The listing builds one solid part. Answer for the finished solid, in the listing's coordinates (mm). A direction names the side the tool comes from. Give positions to 0.01 mm unless a question says otherwise; leave off trailing zeros. Write each loop counter-clockwise with the first axis right and the second up, starting at its lowest first coordinate (ties: lowest second). Pieces come first, ordered by that corner, then holes. Notation, with made-up numbers: (77.5, 76.5) - (89.5, 76.5) arc R29 cw to (89.5, 108.5) - close; hole circle Ø5 at (16, -2). An arc over 180 degrees is marked (long way). Use a Markdown table: item, result. Add a question column.
from build123d import *

# Parameters (mm, degrees)
SKETCH_1_W          = 241
SKETCH_1_H          = 92
EXTRUDE_1_DEPTH     = 2
FILLET_1_R          = 5
FILLET_2_R          = 11
CUT_EXTRUDE_1_REACH = 130.997
SKETCH_3_R          = 1
SKETCH_4_R          = 2
CUT_EXTRUDE_2_DEPTH = 1.3
EXTRUDE_START       = 2
EXTRUDE_2_DEPTH     = 2
CHAMFER_1_SIZE      = 0.174977327
CHAMFER_1_SIZE_2    = 2
SKETCH_6_W          = 5
SKETCH_6_H          = 85
EXTRUDE_3_DEPTH     = 6.3
CUT_EXTRUDE_3_REACH = 131.135
SKETCH_7_W          = 21
SKETCH_7_H          = 60
EXTRUDE_START_2     = -28.5
EXTRUDE_4_DEPTH     = 2
CHAMFER_2_SIZE      = 3
CHAMFER_2_SIZE2     = 1.732050808


with BuildPart() as part:
    # 草图1 → 凸台-拉伸1 (new body)
    with BuildSketch(Plane.XY):
        Rectangle(SKETCH_1_W, SKETCH_1_H)
    extrude(amount=EXTRUDE_1_DEPTH)

    # 圆角1
    fillet_1_edges = [part.edges().sort_by_distance(p)[0] for p in [
        (-120.5, -46, 1),
    ]]
    fillet(fillet_1_edges, radius=FILLET_1_R)

    # 圆角2
    fillet_2_edges = [part.edges().sort_by_distance(p)[0] for p in [
        (120.5, -46, 1),
        (-120.5, 46, 1),
        (120.5, 46, 1),
    ]]
    fillet(fillet_2_edges, radius=FILLET_2_R)

    # 草图3 → 切除-拉伸1 (cut, up to next)
    with BuildSketch(Plane.XY.offset(2), mode=Mode.PRIVATE) as cut_extrude_1_sk1:
        with Locations((-19.5, -41)):
            Circle(SKETCH_3_R)
    cut_extrude_1_tool1 = extrude(cut_extrude_1_sk1.sketch, amount=-CUT_EXTRUDE_1_REACH, mode=Mode.PRIVATE) & part.part
    # 草图3 → 切除-拉伸1 (cut, up to next)
    with BuildSketch(Plane.XY.offset(2), mode=Mode.PRIVATE) as cut_extrude_1_sk2:
        with Locations((-74.5, -40)):
            Circle(SKETCH_3_R)
    cut_extrude_1_tool2 = extrude(cut_extrude_1_sk2.sketch, amount=-CUT_EXTRUDE_1_REACH, mode=Mode.PRIVATE) & part.part
    # 草图3 → 切除-拉伸1 (cut, up to next)
    with BuildSketch(Plane.XY.offset(2), mode=Mode.PRIVATE) as cut_extrude_1_sk3:
        with Locations((-113.5, 39)):
            Circle(SKETCH_3_R)
    cut_extrude_1_tool3 = extrude(cut_extrude_1_sk3.sketch, amount=-CUT_EXTRUDE_1_REACH, mode=Mode.PRIVATE) & part.part
    # 草图3 → 切除-拉伸1 (cut, up to next)
    with BuildSketch(Plane.XY.offset(2), mode=Mode.PRIVATE) as cut_extrude_1_sk4:
        with Locations((0, 39)):
            Circle(SKETCH_3_R)
    cut_extrude_1_tool4 = extrude(cut_extrude_1_sk4.sketch, amount=-CUT_EXTRUDE_1_REACH, mode=Mode.PRIVATE) & part.part
    # 草图3 → 切除-拉伸1 (cut, up to next)
    with BuildSketch(Plane.XY.offset(2), mode=Mode.PRIVATE) as cut_extrude_1_sk5:
        with Locations((113.5, -39)):
            Circle(SKETCH_3_R)
    cut_extrude_1_tool5 = extrude(cut_extrude_1_sk5.sketch, amount=-CUT_EXTRUDE_1_REACH, mode=Mode.PRIVATE) & part.part
    # 草图3 → 切除-拉伸1 (cut, up to next)
    with BuildSketch(Plane.XY.offset(2), mode=Mode.PRIVATE) as cut_extrude_1_sk6:
        with Locations((113.5, 39)):
            Circle(SKETCH_3_R)
    cut_extrude_1_tool6 = extrude(cut_extrude_1_sk6.sketch, amount=-CUT_EXTRUDE_1_REACH, mode=Mode.PRIVATE) & part.part
    add(cut_extrude_1_tool1.solids().sort_by_distance((-19.5, -41, 2))[0], mode=Mode.SUBTRACT)
    add(cut_extrude_1_tool2.solids().sort_by_distance((-74.5, -40, 2))[0], mode=Mode.SUBTRACT)
    add(cut_extrude_1_tool3.solids().sort_by_distance((-113.5, 39, 2))[0], mode=Mode.SUBTRACT)
    add(cut_extrude_1_tool4.solids().sort_by_distance((0, 39, 2))[0], mode=Mode.SUBTRACT)
    add(cut_extrude_1_tool5.solids().sort_by_distance((113.5, -39, 2))[0], mode=Mode.SUBTRACT)
    add(cut_extrude_1_tool6.solids().sort_by_distance((113.5, 39, 2))[0], mode=Mode.SUBTRACT)

    # 草图4 → 切除-拉伸2 (cut)
    with BuildSketch(Plane(origin=(0, 0, 0), x_dir=(-1, 0, 0), z_dir=(0, 0, -1))):
        with Locations((74.5, -40)):
            Circle(SKETCH_4_R)
        with Locations((19.5, -41)):
            Circle(SKETCH_4_R)
        with Locations((-113.5, -39)):
            Circle(SKETCH_4_R)
        with Locations((-113.5, 39)):
            Circle(SKETCH_4_R)
        with Locations((0, 39)):
            Circle(SKETCH_4_R)
        with Locations((113.5, 39)):
            Circle(SKETCH_4_R)
    extrude(amount=-CUT_EXTRUDE_2_DEPTH, mode=Mode.SUBTRACT)

    # 草图5 → 凸台-拉伸2 (add)
    with BuildSketch(Plane.XY.offset(2).offset(EXTRUDE_START)):
        with BuildLine():
            ThreePointArc((-120.5, -41), (-119.035533906, -44.535533906), (-115.5, -46))
            Line((-115.5, -46), (109.5, -46))
            ThreePointArc((109.5, -46), (117.278174593, -42.778174593), (120.5, -35))
            Line((120.5, -35), (120.5, 35))
            ThreePointArc((120.5, 35), (117.278174593, 42.778174593), (109.5, 46))
            Line((109.5, 46), (-109.5, 46))
            ThreePointArc((-109.5, 46), (-117.278174593, 42.778174593), (-120.5, 35))
            Line((-120.5, 35), (-120.5, -41))
        make_face()
        with BuildLine():
            Line((109.5, -44.7), (-115.5, -44.7))
            ThreePointArc((-115.5, -44.7), (-118.11629509, -43.61629509), (-119.2, -41))
            Line((-119.2, -41), (-119.2, 35))
            ThreePointArc((-119.2, 35), (-116.358935778, 41.858935778), (-109.5, 44.7))
            Line((-109.5, 44.7), (109.5, 44.7))
            ThreePointArc((109.5, 44.7), (116.358935778, 41.858935778), (119.2, 35))
            Line((119.2, 35), (119.2, -35))
            ThreePointArc((119.2, -35), (116.358935778, -41.858935778), (109.5, -44.7))
        make_face(mode=Mode.SUBTRACT)
    extrude(amount=-EXTRUDE_2_DEPTH)

    # 倒角1
    # the kernel refuses this chamfer: 2, 0.174977327 mm, written as the material it takes off along each edge
    with BuildSketch(Plane(origin=(-109.5, 44.7, 4), x_dir=(0, 0.9159861691531133, 0.40120984275090293), z_dir=(1, 0, 0))) as chamfer_1_piece_1_section:
        Polygon((CHAMFER_1_SIZE * 0.915986169425, -CHAMFER_1_SIZE * 0.40120984287), (-CHAMFER_1_SIZE_2 * 0.401209842751, -CHAMFER_1_SIZE_2 * 0.915986169153), (0, 0), align=None)
    chamfer_1_piece_1 = extrude(amount=219, mode=Mode.PRIVATE)
    chamfer_1_piece_1 = split(chamfer_1_piece_1, bisect_by=Plane(origin=(0, 44.735649873, 2), z_dir=(0, 0, 1)), keep=Keep.TOP, mode=Mode.PRIVATE)
    add(chamfer_1_piece_1, mode=Mode.SUBTRACT)
    with BuildSketch(Plane(origin=(109.5, 35, 4), x_dir=(0, 1, 0), z_dir=(-1, 0, 0))) as chamfer_1_piece_2_section:
        Polygon((9.7 + CHAMFER_1_SIZE, 0), (9.7, CHAMFER_1_SIZE_2), (9.7, 0), align=None)
    chamfer_1_piece_2 = revolve(axis=Axis((109.5, 35, 4), (0, 0, -1)), revolution_arc=90, mode=Mode.PRIVATE)
    chamfer_1_piece_2 = split(chamfer_1_piece_2, bisect_by=Plane(origin=(116.41200817, 41.91200817, 2), z_dir=(0, 0, 1)), keep=Keep.TOP, mode=Mode.PRIVATE)
    add(chamfer_1_piece_2, mode=Mode.SUBTRACT)
    with BuildSketch(Plane(origin=(-109.5, 35, 4), x_dir=(-1, 0, 0), z_dir=(0, -1, 0))) as chamfer_1_piece_3_section:
        Polygon((9.7 + CHAMFER_1_SIZE, 0), (9.7, CHAMFER_1_SIZE_2), (9.7, 0), align=None)
    chamfer_1_piece_3 = revolve(axis=Axis((-109.5, 35, 4), (0, 0, -1)), revolution_arc=90, mode=Mode.PRIVATE)
    chamfer_1_piece_3 = split(chamfer_1_piece_3, bisect_by=Plane(origin=(-116.412008168, 41.912008168, 2), z_dir=(0, 0, 1)), keep=Keep.TOP, mode=Mode.PRIVATE)
    add(chamfer_1_piece_3, mode=Mode.SUBTRACT)
    with BuildSketch(Plane(origin=(119.2, 35, 4), x_dir=(0.9159861691531133, 0, 0.40120984275090293), z_dir=(0, -1, 0))) as chamfer_1_piece_4_section:
        Polygon((CHAMFER_1_SIZE * 0.915986169425, -CHAMFER_1_SIZE * 0.40120984287), (-CHAMFER_1_SIZE_2 * 0.401209842751, -CHAMFER_1_SIZE_2 * 0.915986169153), (0, 0), align=None)
    chamfer_1_piece_4 = extrude(amount=70, mode=Mode.PRIVATE)
    chamfer_1_piece_4 = split(chamfer_1_piece_4, bisect_by=Plane(origin=(119.235649873, 0, 2), z_dir=(0, 0, 1)), keep=Keep.TOP, mode=Mode.PRIVATE)
    add(chamfer_1_piece_4, mode=Mode.SUBTRACT)
    with BuildSketch(Plane(origin=(-119.2, -41, 4), x_dir=(-0.9159861691531133, 0, 0.40120984275090293), z_dir=(0, 1, 0))) as chamfer_1_piece_5_section:
        Polygon((CHAMFER_1_SIZE * 0.915986169425, -CHAMFER_1_SIZE * 0.40120984287), (-CHAMFER_1_SIZE_2 * 0.401209842751, -CHAMFER_1_SIZE_2 * 0.915986169153), (0, 0), align=None)
    chamfer_1_piece_5 = extrude(amount=76, mode=Mode.PRIVATE)
    chamfer_1_piece_5 = split(chamfer_1_piece_5, bisect_by=Plane(origin=(-119.235649873, -3, 2), z_dir=(0, 0, 1)), keep=Keep.TOP, mode=Mode.PRIVATE)
    add(chamfer_1_piece_5, mode=Mode.SUBTRACT)
    with BuildSketch(Plane(origin=(109.5, -35, 4), x_dir=(1, 0, 0), z_dir=(0, 1, 0))) as chamfer_1_piece_6_section:
        Polygon((9.7 + CHAMFER_1_SIZE, 0), (9.7, CHAMFER_1_SIZE_2), (9.7, 0), align=None)
    chamfer_1_piece_6 = revolve(axis=Axis((109.5, -35, 4), (0, 0, -1)), revolution_arc=90, mode=Mode.PRIVATE)
    chamfer_1_piece_6 = split(chamfer_1_piece_6, bisect_by=Plane(origin=(116.41200817, -41.91200817, 2), z_dir=(0, 0, 1)), keep=Keep.TOP, mode=Mode.PRIVATE)
    add(chamfer_1_piece_6, mode=Mode.SUBTRACT)
    with BuildSketch(Plane(origin=(-115.5, -41, 4), x_dir=(0, -1, 0), z_dir=(1, 0, 0))) as chamfer_1_piece_7_section:
        Polygon((3.7 + CHAMFER_1_SIZE, 0), (3.7, CHAMFER_1_SIZE_2), (3.7, 0), align=None)
    chamfer_1_piece_7 = revolve(axis=Axis((-115.5, -41, 4), (0, 0, -1)), revolution_arc=90, mode=Mode.PRIVATE)
    chamfer_1_piece_7 = split(chamfer_1_piece_7, bisect_by=Plane(origin=(-118.172444307, -43.672444307, 2), z_dir=(0, 0, 1)), keep=Keep.TOP, mode=Mode.PRIVATE)
    add(chamfer_1_piece_7, mode=Mode.SUBTRACT)
    with BuildSketch(Plane(origin=(109.5, -44.7, 4), x_dir=(0, -0.9159861691531133, 0.40120984275090293), z_dir=(-1, 0, 0))) as chamfer_1_piece_8_section:
        Polygon((CHAMFER_1_SIZE * 0.915986169425, -CHAMFER_1_SIZE * 0.40120984287), (-CHAMFER_1_SIZE_2 * 0.401209842751, -CHAMFER_1_SIZE_2 * 0.915986169153), (0, 0), align=None)
    chamfer_1_piece_8 = extrude(amount=225, mode=Mode.PRIVATE)
    chamfer_1_piece_8 = split(chamfer_1_piece_8, bisect_by=Plane(origin=(-3, -44.735649873, 2), z_dir=(0, 0, 1)), keep=Keep.TOP, mode=Mode.PRIVATE)
    add(chamfer_1_piece_8, mode=Mode.SUBTRACT)

    # 草图6 → 凸台-拉伸3 (add)
    with BuildSketch(Plane.XY.offset(2)):
        with Locations((26.5, 0)):
            Rectangle(SKETCH_6_W, SKETCH_6_H)
    extrude(amount=EXTRUDE_3_DEPTH)

    # 草图7 → 切除-拉伸3 (cut, up to next)
    with BuildSketch(Plane.XY.offset(2), mode=Mode.PRIVATE) as cut_extrude_3_sk1:
        with Locations((-104.5, -9)):
            Rectangle(SKETCH_7_W, SKETCH_7_H)
    cut_extrude_3_tool1 = extrude(cut_extrude_3_sk1.sketch, amount=-CUT_EXTRUDE_3_REACH, mode=Mode.PRIVATE) & part.part
    add(cut_extrude_3_tool1.solids().sort_by_distance((-104.5, -9, 2))[0], mode=Mode.SUBTRACT)

    # 草图8 → 凸台-拉伸4 (add)
    with BuildSketch(Plane.ZY.offset(120.5).offset(EXTRUDE_START_2)):
        with BuildLine():
            Line((2, -21), (2, -42.5))
            Line((2, -42.5), (39.5, -42.5))
            Line((39.5, -42.5), (39.5, -40.556496954))
            ThreePointArc((39.5, -40.556496954), (19.774984647, -36.291232599), (6.605059959, -21))
            Line((6.605059959, -21), (2, -21))
        make_face()
        with BuildLine():
            Line((2, -14), (4.646172482, -14))
            ThreePointArc((4.646172482, -14), (5.952882138, 1.25832385), (14.25, 14.130067012))
            Line((14.25, 14.130067012), (14.25, 27))
            Line((14.25, 27), (12.5, 27))
            Line((12.5, 27), (12.5, 42.479565739))
            Line((12.5, 42.479565739), (2, 42.479565739))
            Line((2, 42.479565739), (2, -14))
        make_face()
    extrude(amount=EXTRUDE_4_DEPTH)

    # 倒角2
    chamfer_2_edges = [part.edges().sort_by_distance(p)[0] for p in [
        (-104.5, -39, 0),
        (-115, -9, 0),
        (-104.5, 21, 0),
        (-94, -9, 0),
    ]]
    chamfer_2_side = [part.faces().sort_by_distance(p)[0] for p in [
        (6.21588018, 0.505356203, 0),
    ]]
    chamfer(chamfer_2_edges, length=CHAMFER_2_SIZE, length2=CHAMFER_2_SIZE2, reference=chamfer_2_side[0])


solid = part.part
1. The part is cut by section A-A (y = -17). Give the vertices of the cut face in (x, z), and give its area (3 significant figures).
2. The part is cut by section D-D (y = 8.5). Give the vertices of the cut face in (x, z), and give its area (3 significant figures).
3. Which of the six approach directions +Z, -Z, +X, -X, +Y, -Y give full straight-line access (tool end or side, diameter ignored) to faces 1 (the cylindrical face through (-19.066, -42.952, 0.641)), 2 (the flat face through (-120.5, -2, 2)), 3 (the flat face through (-92, -36, 12))?
4. Given P1, Ø1.6, axis at x = 113.5, y = 39, coming from the -Z side; P2, Ø5, axis at x = -19.5, y = -41, coming from the +Z side; P3, Ø1, axis at x = -92.5, y = 20.5, coming from the +Z side; P4, Ø2, axis at x = -92.5, z = 5.5, coming from the +Y side, each flat-ended and moving along its own axis, determine where each tip first touches the part or whether it passes through.
5. Consider L1, parallel to X at y = -31, z = 4.5; L2, parallel to Y at x = -74.5, z = 1; L3, parallel to Y at x = -82.5, z = 2.5. Determine where each line is inside the solid, lowest interval first. Write a range as [from, to].
6. The part is cut by section B-B (x = -102). Give the vertices of the cut face in (y, z), and give its area (3 significant figures).
7. The part is cut by section C-C (x = 5). Give the vertices of the cut face in (y, z).
8. For a pull along Y with two mould halves and no side action, classify faces 4 (the flat face through (-2, 1, 0)), 5 (the flat face through (-5, -46, 2)), 6 (the flat face through (-20.4, -41.9, 1.3)) as released by +Y, released by -Y, zero draft, split by the parting line, or undercut.
Check values:
| question | item | result |
|---|---|---|
| 1 | outline | (-120.5, 0) - (-118, 0) - (-115, 1.73) - (-115, 2) - (-119.2, 2) - (-119.37, 4) - (-120.5, 4) - close; (-94, 1.73) - (-91, 0) - (120.5, 0) - (120.5, 4) - (119.37, 4) - (119.2, 2) - (29, 2) - (29, 8.3) - (24, 8.3) - (24, 2) - (-94, 2) - close |
| 1 | area | 471 mm2 |
| 2 | outline | (-120.5, 0) - (-118, 0) - (-115, 1.73) - (-115, 2) - (-119.2, 2) - (-119.37, 4) - (-120.5, 4) - close; (-94, 1.73) - (-91, 0) - (120.5, 0) - (120.5, 4) - (119.37, 4) - (119.2, 2) - (29, 2) - (29, 8.3) - (24, 8.3) - (24, 2) - (-92, 2) - (-92, 9.51) - (-94, 9.51) - close |
| 2 | area | 486 mm2 |
| 3 | face 1 | -Z |
| 3 | face 2 | +Z, -Z, -X, +Y, -Y |
| 3 | face 3 | +Z |
| 4 | P1 | passes through |
| 4 | P2 | stops at z = 2 |
| 4 | P3 | stops at z = 14.25 |
| 4 | P4 | stops at y = 42.48 |
| 5 | L1 | x = [-94, -92], [24, 29] |
| 5 | L2 | y = [-46, -42], [-38, 46] |
| 5 | L3 | y = [-46, -44.74], [44.74, 46] |
| 6 | outline | (-46, 0) - (-42, 0) - (-39, 1.73) - (-39, 2) - (-44.7, 2) - (-44.87, 4) - (-46, 4) - close; (21, 1.73) - (24, 0) - (46, 0) - (46, 4) - (44.87, 4) - (44.7, 2) - (21, 2) - close |
| 6 | area | 63.7 mm2 |
| 7 | outline | (-46, 0) - (46, 0) - (46, 4) - (44.87, 4) - (44.7, 2) - (-44.7, 2) - (-44.87, 4) - (-46, 4) - close |
| 8 | face 4 | zero draft |
| 8 | face 5 | released by -Y |
| 8 | face 6 | undercut |
